Design review of the part built by this model. Coordinates are the model's own, in mm. A direction names the side the tool comes from. Give positions to 0.01 mm unless a question says otherwise; leave off trailing zeros. Loops run counter-clockwise (first coordinate to the right, second up) from the corner with the lowest first, then second, coordinate; pieces in that order, holes last. Notation, with made-up numbers: M 62,28.5 L 88,28.5 A19 ccw 88,55.5 Z; hole C 63,84 d2. An arc over 180 degrees is marked long. Use a Markdown table: item, result. Add a question column.
(1) Add section D-D, the plane y = 2.5. State how many separate pieces and enclosed holes the cut face has, then the cut area to 3 significant figures.
(2) Insertion check: pin 1 Ø12 at (x, z) = (-57, 68.5) entering from +Y; pin 2 Ø4 at (y, z) = (1.5, -22) entering from -X. Each pin has a flat end and moves straight along its axis. Give the tip position at first contact, or say it passes through.
(3) For probe 1 along X at (y, z) = (-0.75, -70); probe 2 along Z at (x, y) = (65, 3.5); probe 3 along X at (y, z) = (-0.5, -37), list the stretches that pass through material, from the lowest coordinate up.
(4) Add section C-C, the plane x = -42. Give the boundary of the cut face in (y, z).
(5) Add section B-B, the plane z = -48. Give the boundary of the cut face in (x, y).
(6) For faces 4 (the face through (72.15, 0.06, -43.01)), 5 (the face through (-59, -1, 74)), 6 (the face through (-35, 0, 0)), list the 3-axis set-ups (+Z, -Z, +X, -X, +Y, -Y) from which the entire face can be reached by the end or side of a thin tool; tool diameter is ignored.
(7) Draft analysis for pull direction Z (two halves, no side actions). For faces 1 (the face through (-1, 0, -90)), 2 (the face through (-22.52, 0.06, 70.33)), 3 (the face through (75, 0, 60)), state which applies: pulls with the +Z half, pulls with the -Z half, needs draft (parallel to the pull), parting line crosses it, or undercut.
(8) Add section A-A, the plane x = 55. Give the boundary of the cut face in (y, z), then the cut area to 3 significant figures.
```python
from build123d import *

# Parameters (mm, degrees)
SKETCH2_W               = 150
SKETCH2_H               = 180
BOSS_EXTRUDE1_DEPTH     = 4
FILLET1_SIZE            = 10
FILLET1_SIZE_2          = 20
FILLET2_SIZE            = 10
FILLET2_SIZE_2          = 20
SKETCH3_R               = 9.65
CUT_EXTRUDE1_DEPTH      = 5
SKETCH7_R               = 5
CUT_EXTRUDE4_DEPTH      = 118.426572949
MIRROR2_COPY_1_SKETCH_R = 9.65
MIRROR2_COPY_1_DEPTH    = 5
MIRROR2_COPY_2_SKETCH_R = 5
MIRROR2_COPY_2_DEPTH    = 118.426572949
SKETCH4_W               = 80
SKETCH4_H               = 80
CUT_EXTRUDE2_DEPTH      = 118.426572949
FILLET3_R               = 10
SKETCH6_R               = 2.5
CUT_EXTRUDE3_DEPTH      = 118.426572949


with BuildPart() as part:
    # Sketch2 → Boss-Extrude1 (new, symmetric)
    with BuildSketch(Plane(origin=(0, 0, 0), x_dir=(1, 0, 0), z_dir=(0, 1, 0))):
        Rectangle(SKETCH2_W, SKETCH2_H)
    extrude(amount=BOSS_EXTRUDE1_DEPTH, both=True)

    # Fillet1
    # an asymmetric fillet: 20, 10 mm, written as the material it takes off along each edge
    with BuildSketch(Plane(origin=(-75, -54, -90), x_dir=(1, 0, 0), z_dir=(0, 1, 0))) as fillet1_piece_1:
        with BuildLine():
            Bezier((FILLET1_SIZE, 0), (0, 0), (0, -FILLET1_SIZE_2), weights=[1, 0.707106781, 1])
            Line((0, -FILLET1_SIZE_2), (0, 0))
            Line((0, 0), (FILLET1_SIZE, 0))
        make_face()
    extrude(amount=108, mode=Mode.SUBTRACT)
    with BuildSketch(Plane(origin=(75, 54, 90), x_dir=(-1, 0, 0), z_dir=(0, -1, 0))) as fillet1_piece_2:
        with BuildLine():
            Bezier((FILLET1_SIZE, 0), (0, 0), (0, FILLET1_SIZE_2), weights=[1, 0.707106781, 1])
            Line((0, FILLET1_SIZE_2), (0, 0))
            Line((0, 0), (FILLET1_SIZE, 0))
        make_face()
    extrude(amount=108, mode=Mode.SUBTRACT)

    # Fillet2
    # an asymmetric fillet: 20, 10 mm, written as the material it takes off along each edge
    with BuildSketch(Plane(origin=(75, 54, -90), x_dir=(-1, 0, 0), z_dir=(0, -1, 0))) as fillet2_piece_1:
        with BuildLine():
            Bezier((FILLET2_SIZE, 0), (0, 0), (0, -FILLET2_SIZE_2), weights=[1, 0.707106781, 1])
            Line((0, -FILLET2_SIZE_2), (0, 0))
            Line((0, 0), (FILLET2_SIZE, 0))
        make_face()
    extrude(amount=108, mode=Mode.SUBTRACT)
    with BuildSketch(Plane(origin=(-75, -54, 90), x_dir=(0, 0, -1), z_dir=(0, 1, 0))) as fillet2_piece_2:
        with BuildLine():
            Bezier((FILLET2_SIZE_2, 0), (0, 0), (0, -FILLET2_SIZE), weights=[1, 0.707106781, 1])
            Line((0, -FILLET2_SIZE), (0, 0))
            Line((0, 0), (FILLET2_SIZE_2, 0))
        make_face()
    extrude(amount=108, mode=Mode.SUBTRACT)

    # Sketch3 → Cut-Extrude1 (cut)
    with BuildSketch(Plane(origin=(0, 4, 0), x_dir=(1, 0, 0), z_dir=(0, 1, 0))):
        with Locations(Location((-55, -70, 0), (0, 0, 270))):
            Circle(SKETCH3_R)
    cut_extrude1 = extrude(amount=-CUT_EXTRUDE1_DEPTH, mode=Mode.SUBTRACT)

    # Sketch7 → Cut-Extrude4 (cut, through all)
    with BuildSketch(Plane(origin=(0, 4, 0), x_dir=(1, 0, 0), z_dir=(0, 1, 0))):
        with Locations(Location((-55, -70, 0), (0, 0, 270))):
            Circle(SKETCH7_R)
    cut_extrude4 = extrude(amount=-CUT_EXTRUDE4_DEPTH, mode=Mode.SUBTRACT)

    # Mirror1: Cut-Extrude1, Cut-Extrude4 across plane
    add(cut_extrude1.mirror(Plane.XY), mode=Mode.SUBTRACT)
    add(cut_extrude4.mirror(Plane.XY), mode=Mode.SUBTRACT)

    # Mirror2: Cut-Extrude1, Cut-Extrude4 across plane
    add(cut_extrude1.mirror(Plane(origin=(0, 0, 0), x_dir=(0, 0, 1), z_dir=(1, 0, 0))), mode=Mode.SUBTRACT)
    add(cut_extrude4.mirror(Plane(origin=(0, 0, 0), x_dir=(0, 0, 1), z_dir=(1, 0, 0))), mode=Mode.SUBTRACT)

    # Mirror2 copy 1 sketch → Mirror2 copy 1 (cut)
    with BuildSketch(Plane(origin=(0, 4, 0), x_dir=(-1, 0, 0), z_dir=(0, 1, 0))):
        with Locations(Location((-55, -70, 0), (0, 0, 270))):
            Circle(MIRROR2_COPY_1_SKETCH_R)
    extrude(amount=-MIRROR2_COPY_1_DEPTH, mode=Mode.SUBTRACT)

    # Mirror2 copy 2 sketch → Mirror2 copy 2 (cut, through all)
    with BuildSketch(Plane(origin=(0, 4, 0), x_dir=(-1, 0, 0), z_dir=(0, 1, 0))):
        with Locations(Location((-55, -70, 0), (0, 0, 270))):
            Circle(MIRROR2_COPY_2_SKETCH_R)
    extrude(amount=-MIRROR2_COPY_2_DEPTH, mode=Mode.SUBTRACT)

    # Sketch4 → Cut-Extrude2 (cut, through all)
    with BuildSketch(Plane(origin=(0, 4, 0), x_dir=(1, 0, 0), z_dir=(0, 1, 0))):
        with Locations((-75, 0)):
            Rectangle(SKETCH4_W, SKETCH4_H)
    cut_extrude2 = extrude(amount=-CUT_EXTRUDE2_DEPTH, mode=Mode.SUBTRACT)

    # Mirror3: Cut-Extrude2 across plane
    add(cut_extrude2.mirror(Plane(origin=(0, 0, 0), x_dir=(0, 0, 1), z_dir=(1, 0, 0))), mode=Mode.SUBTRACT)

    # Fillet3
    fillet3_edges = [part.edges().sort_by_distance(p)[0] for p in [
        (75, 0, -40),
        (75, 0, 40),
        (-75, 0, -40),
        (-75, 0, 40),
        (-35, 0, -40),
        (-35, 0, 40),
        (35, 0, 40),
        (35, 0, -40),
    ]]
    fillet(fillet3_edges, radius=FILLET3_R)

    # Sketch6 → Cut-Extrude3 (cut, through all)
    with BuildSketch(Plane(origin=(0, 4, 0), x_dir=(1, 0, 0), z_dir=(0, 1, 0))):
        with Locations(Location((-25, 81, 0), (0, 0, 270))):
            Circle(SKETCH6_R)
        with Locations(Location((25, 81, 0), (0, 0, 270))):
            Circle(SKETCH6_R)
        with Locations(Location((0, 81, 0), (0, 0, 270))):
            Circle(SKETCH6_R)
        with Locations(Location((-25, 70, 0), (0, 0, 270))):
            Circle(SKETCH6_R)
        with Locations(Location((0, 70, 0), (0, 0, 270))):
            Circle(SKETCH6_R)
        with Locations(Location((25, 70, 0), (0, 0, 270))):
            Circle(SKETCH6_R)
        with Locations(Location((-25, 59, 0), (0, 0, 270))):
            Circle(SKETCH6_R)
        with Locations(Location((0, 59, 0), (0, 0, 270))):
            Circle(SKETCH6_R)
        with Locations(Location((25, 59, 0), (0, 0, 270))):
            Circle(SKETCH6_R)
        with Locations(Location((-25, 48, 0), (0, 0, 270))):
            Circle(SKETCH6_R)
        with Locations(Location((0, 48, 0), (0, 0, 270))):
            Circle(SKETCH6_R)
        with Locations(Location((25, 48, 0), (0, 0, 270))):
            Circle(SKETCH6_R)
        with Locations(Location((-25, 37, 0), (0, 0, 270))):
            Circle(SKETCH6_R)
        with Locations(Location((0, 37, 0), (0, 0, 270))):
            Circle(SKETCH6_R)
        with Locations(Location((25, 37, 0), (0, 0, 270))):
            Circle(SKETCH6_R)
    cut_extrude3 = extrude(amount=-CUT_EXTRUDE3_DEPTH, mode=Mode.SUBTRACT)

    # Mirror4: Cut-Extrude3 across plane
    add(cut_extrude3.mirror(Plane.XY), mode=Mode.SUBTRACT)


solid = part.part
```
Established:
| question | item | result |
|---|---|---|
| 1 | separate pieces | 1 |
| 1 | enclosed holes | 34 |
| 1 | area | 18,700 mm^2 |
| 2 | pin 1 | y = -1 |
| 2 | pin 2 | x = -35 |
| 3 | probe 1 | -75 to -64.65, -45.35 to -27.5, -22.5 to -2.5, 2.5 to 22.5, 27.5 to 45.35, 64.65 to 75 |
| 3 | probe 2 | -90 to -40, 40 to 90 |
| 3 | probe 3 | -37.86 to -27.5, -22.5 to -2.5, 2.5 to 22.5, 27.5 to 37.86 |
| 4 | outline | M -4,-90 L 4,-90 L 4,-39.54 L -4,-39.54 Z; M -4,39.54 L 4,39.54 L 4,90 L -4,90 Z |
| 5 | outline | M -74.8,-4 L -27.5,-4 L -27.5,4 L -74.8,4 Z; M -22.5,-4 L -2.5,-4 L -2.5,4 L -22.5,4 Z; M 2.5,-4 L 22.5,-4 L 22.5,4 L 2.5,4 Z; M 27.5,-4 L 74.8,-4 L 74.8,4 L 27.5,4 Z |
| 6 | face 4 | +X, +Y, -Y |
| 6 | face 5 | +Y |
| 6 | face 6 | -X, +Y, -Y |
| 7 | face 1 | pulls with the -Z half |
| 7 | face 2 | undercut |
| 7 | face 3 | needs draft |
| 8 | outline | M -4,-90 L 4,-90 L 4,-79.65 L -1,-79.65 L -1,-75 L -4,-75 Z; M -4,-65 L -1,-65 L -1,-60.35 L 4,-60.35 L 4,-40 L -4,-40 Z; M -4,40 L 4,40 L 4,60.35 L -1,60.35 L -1,65 L -4,65 Z; M -4,75 L -1,75 L -1,79.65 L 4,79.65 L 4,90 L -4,90 Z |
| 8 | area | 547 mm^2 |
